For this review, use the dimensioned drawing (mm, ordinates from the lowest corner) and the shaded views. A direction names the side the tool comes from. Round coordinates to 2 decimals unless told otherwise and drop trailing zeros. Write each loop counter-clockwise with the first axis right and the second up, starting at its lowest first coordinate (ties: lowest second). Pieces come first, ordered by that corner, then holes. Notation, with made-up numbers: (66.5, 0) -> (78.5, 0) arc R24 cw to (78.5, 16) -> close; hole circle Ø2 at (8, 4.5). An arc over 180 degrees is marked (long way). Answer in a Markdown table with one row per item. Add a question column.
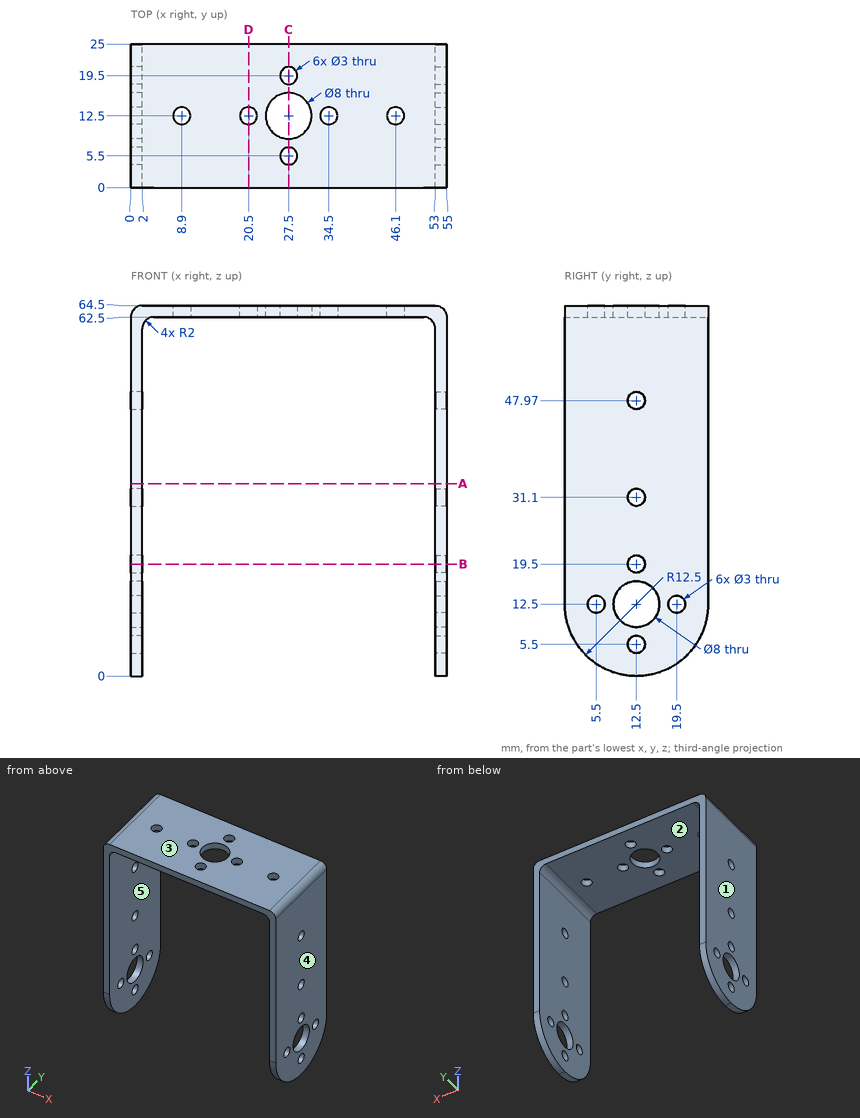
1. We need section C-C (x = 27.5). Write out the cut boundary in (y, z).
2. Clearance check with flat-ended pins moving along their axes: pin 1 Ø2.5 at (y, z) = (12.5, 19.5) entering from +X (1 decimal); pin 2 Ø5 at (x, y) = (20, 22) entering from -Z. State where each tip first meets the part, or that it passes through.
3. Tool access review of the marked faces 1 and 2: name each direction out of +Z, -Z, +X, -X, +Y, -Y from which nothing blocks a thin tool from reaching the whole face with its end or side.
4. We need section A-A (z = 33.5). Write out the cut boundary in (x, y).
5. The part is to be moulded in two halves that separate along X. For the marked faces 3, 4 and 5, say which applies: pulls with the +X half, pulls with the -X half, needs draft (parallel to the pull), parting line crosses it, or undercut.
6. We need section D-D (x = 20.5). Write out the cut boundary in (y, z), plus the area to 3 significant figures.
7. We need section B-B (z = 19.5). Write out the cut boundary in (x, y), plus the area to 3 significant figures.
8. For L1, parallel to X at y = 3.75, z = 51; L2, parallel to Y at x = 1.5, z = 12.5; L3, parallel to Y at x = 53.55, z = 47.97, list the stretches that pass through material, from the lowest coordinate up. Write a range as [from, to].
Response:
| question | item | result |
|---|---|---|
| 1 | outline | (0, 62.5) -> (4, 62.5) -> (4, 64.5) -> (0, 64.5) -> close; (7, 62.5) -> (8.5, 62.5) -> (8.5, 64.5) -> (7, 64.5) -> close; (16.5, 62.5) -> (18, 62.5) -> (18, 64.5) -> (16.5, 64.5) -> close; (21, 62.5) -> (25, 62.5) -> (25, 64.5) -> (21, 64.5) -> close |
| 2 | pin 1 | through |
| 2 | pin 2 | z = 62.5 |
| 3 | face 1 | +Z, -Z, -X, +Y, -Y |
| 3 | face 2 | -Z, +Y, -Y |
| 4 | outline | (0, 0) -> (2, 0) -> (2, 25) -> (0, 25) -> close; (53, 0) -> (55, 0) -> (55, 25) -> (53, 25) -> close |
| 5 | face 3 | needs draft |
| 5 | face 4 | pulls with the +X half |
| 5 | face 5 | undercut |
| 6 | outline | (0, 62.5) -> (11, 62.5) -> (11, 64.5) -> (0, 64.5) -> close; (14, 62.5) -> (25, 62.5) -> (25, 64.5) -> (14, 64.5) -> close |
| 6 | area | 44.0 mm2 |
| 7 | outline | (0, 0) -> (2, 0) -> (2, 11) -> (0, 11) -> close; (0, 14) -> (2, 14) -> (2, 25) -> (0, 25) -> close; (53, 0) -> (55, 0) -> (55, 11) -> (53, 11) -> close; (53, 14) -> (55, 14) -> (55, 25) -> (53, 25) -> close |
| 7 | area | 88.0 mm2 |
| 8 | L1 | [0, 2], [53, 55] |
| 8 | L2 | [0, 4], [7, 8.5], [16.5, 18], [21, 25] |
| 8 | L3 | [0, 11], [14, 25] |
